from build123d import *

# Parameters (mm, degrees)
F1_DEPTH = 50.8
F2_W     = 14.4103989005
F2_H     = 18.3605216444
F3_DEPTH = 25.4


with BuildPart() as f1:
    # F0 (on Front) → F1 (new body)
    with BuildSketch(Plane.XZ):
        Polygon((0, 43.7689125538), (0, 0), (65.3845146298, 0), (65.3845146298, 43.7689125538), (50.9741157293, 43.7689125538), (50.9741157293, 13.6576220393), (17.4215342849, 13.6576220393), (17.4215342849, 43.7689125538), align=None)
    extrude(amount=F1_DEPTH)

    # F2 (on face) → F3 (cut)
    with BuildSketch(Plane.XY.offset(43.7689125538)):
        with Locations((58.1793151796, -24.6975105256)):
            Rectangle(F2_W, F2_H)
    extrude(amount=-F3_DEPTH, mode=Mode.SUBTRACT)


solid = f1.part
Geometry: final body of the model. Coordinates: model frame, mm. A direction names the side the tool comes from. Give positions to 0.01 mm unless a question says otherwise; leave off trailing zeros. Write each loop counter-clockwise with the first axis right and the second up, starting at its lowest first coordinate (ties: lowest second). Pieces come first, ordered by that corner, then holes. Notation, with made-up numbers: M 44.5,63.25 L 78.5,63.25 A20 ccw 78.5,86.25 Z; hole C 51.5,30.5 d2. An arc over 180 degrees is marked long. Answer in a Markdown table with one row per item. Add a question column.
(1) Reachability of faces 1 (the flat face through (58, -15.517, 31)), 2 (the flat face through (65.385, -25, 17)), 3 (the flat face through (17.422, -25, 29)) from +Z, -Z, +X, -X, +Y, -Y: full face, straight path, thin tool, end or side. Return the list, or none.
(2) Section D-D on x = 57. Return loops of the section in (y, z), and give its area (3 significant figures).
(3) First-contact query: pin 1 (17 mm diameter, centred on x = 36, y = -15.5, fed in from +Z); pin 2 (11.5 mm diameter, centred on x = 55, y = -26.5, fed in from +Z). Flat tips, straight axial feed; report the tip coordinate or a pass-through.
(4) Section B-B on y = -28.5. Return loops of the section in (x, z), and give its area (3 significant figures).
(5) Section C-C on z = 28.5. Return loops of the section in (x, y).
(6) Section A-A on z = 15.5. Return loops of the section in (x, y), and give its area (3 significant figures).
(7) Mould query, pull axis Y, two halves, no side actions, for faces 4 (the flat face through (58, -33.878, 31)), 5 (the flat face through (58, -25, 18.369)), 6 (the flat face through (32, -25, 0)), 7 (the flat face through (32, 0, 12)). Classes: +Y half, -Y half, draft (parallel to the pull), parting line (faces both ways), or undercut.
(8) Ray query, line 1 (X direction, y = -3, z = 29.5); line 2 (Y direction, x = 63, z = 32); line 3 (X direction, y = -26, z = 41). Return the intervals inside material, ascending.
Result set:
| question | item | result |
|---|---|---|
| 1 | face 1 | +Z, +X |
| 1 | face 2 | +Z, -Z, +X, +Y, -Y |
| 1 | face 3 | +Z, +Y, -Y |
| 2 | outline | M -50.8,0 L 0,0 L 0,43.77 L -15.52,43.77 L -15.52,18.37 L -33.88,18.37 L -33.88,43.77 L -50.8,43.77 Z |
| 2 | area | 1,760 mm^2 |
| 3 | pin 1 | stops at z = 13.66 |
| 3 | pin 2 | stops at z = 18.37 |
| 4 | outline | M 0,0 L 65.38,0 L 65.38,18.37 L 50.97,18.37 L 50.97,13.66 L 17.42,13.66 L 17.42,43.77 L 0,43.77 Z |
| 4 | area | 1,490 mm^2 |
| 5 | outline | M 0,-50.8 L 17.42,-50.8 L 17.42,0 L 0,0 Z; M 50.97,-50.8 L 65.38,-50.8 L 65.38,-33.88 L 50.97,-33.88 Z; M 50.97,-15.52 L 65.38,-15.52 L 65.38,0 L 50.97,0 Z |
| 6 | outline | M 0,-50.8 L 17.42,-50.8 L 17.42,0 L 0,0 Z; M 50.97,-50.8 L 65.38,-50.8 L 65.38,0 L 50.97,0 Z |
| 6 | area | 1,620 mm^2 |
| 7 | face 4 | undercut |
| 7 | face 5 | undercut |
| 7 | face 6 | draft |
| 7 | face 7 | +Y half |
| 8 | line 1 | x = 0 to 17.42, 50.97 to 65.38 |
| 8 | line 2 | y = -50.8 to -33.88, -15.52 to 0 |
| 8 | line 3 | x = 0 to 17.42 |
